Work out the finished part from the listing and answer in its coordinate system (mm). Give positions to 0.01 mm unless a question says otherwise; leave off trailing zeros. Loops run counter-clockwise (first coordinate to the right, second up) from the corner with the lowest first, then second, coordinate; pieces in that order, holes last. Notation, with made-up numbers: (-25.75, -33.75) - (23.25, -33.75) arc R28 ccw to (23.25, 0.25) - close; hole circle Ø11 at (85.25, 5.5). An arc over 180 degrees is marked (long way). Use CSV: the item, a comma, the result in double quotes.
Autodesk Inventor part; units mm, degrees
ref_plane "YZ Plane" through (0, 0, 0) normal (1, 0, 0) x (0, 1, 0)
ref_plane "XZ Plane" through (0, 0, 0) normal (0, 1, 0) x (-1, 0, 0)
ref_plane "XY Plane" through (0, 0, 0) normal (0, 0, 1) x (1, 0, 0)
sketch "Sketch1" plane through (0, 0, 0) normal (0, 0, 1) x (1, 0, 0)
  line L0 (-25, 0) -> (25, 0)
  line L1 (25, 0) -> (25, -1190)
  line L2 (25, -1190) -> (-25, -1190)
  line L3 (-25, -1190) -> (-25, 0)
  line L4 (25, -1190) -> (-25, -1153.2713)
  line L5 (25, 0) -> (-25, -68.0668)
  point P0 (0, 0)
  point P1 (0, 0)
  point P2 (25, -1153.2713)
  dimension "d0" = 50
  dimension "d1" = 1190
  dimension "d5" = 53.7
  dimension "d6" = 53.7
extrude "Plate1" add sketch "Sketch1" along normal mid plane 3 contours L1 L4 L3 L5
chamfer "Corner Chamfer1" distance 3 angle 45 1 edges at (25, -1190, 0)
fillet "Corner Round1" radius 6 1 edges at (-25, -1153.2713, 0)
fillet "Corner Round2" radius 6 1 edges at (-25, -68.0668, 0)
chamfer "Corner Chamfer3" distance 3 angle 45 1 edges at (25, 0, 0)
sketch "Sketch3" plane through (0, 0, 1.5) normal (0, 0, 1) x (1, 0, 0)
  line L0 (-1, -188.5) -> (25, -188.5)
  line L1 (25, -188.5) -> (25, -185.5)
  line L2 (25, -185.5) -> (-1, -185.5)
  line L3 (-1, -185.5) -> (-1, -188.5)
  line L4 (25, -3) -> (25, -1187)
  point P0 (0, 0)
  point P1 (25, -187)
  dimension "d18" = 187
  dimension "d19" = 26
  dimension "d20" = 3
extrude "Extrusion1" cut sketch "Sketch3" against normal through all
pattern_linear "Rectangular Pattern1" count 3 spacing 323 along (0, -1, 0) of "Extrusion1"
sketch "Sketch4" plane through (0, 0, -1.5) normal (0, 0, -1) x (-1, 0, 0)
  line L0 (-5.565, -286.9038) -> (3.4627, -286.9038) construction
  line L1 (3.4627, -286.9038) -> (3.4627, -416.417) construction
  line L2 (3.4627, -416.417) -> (-5.565, -416.417) construction
  line L3 (-5.565, -416.417) -> (-5.565, -286.9038) construction
  point P0 (0, 0)
mark "Mark1"
equation "\"d6\" = d5"
equation "\"d2\" = Thickness"
equation "\"BendReliefWidth\" = Thickness"
equation "\"BendReliefDepth\" = 0.5 * Thickness"
equation "\"CornerReliefSize\" = 4 * Thickness"
equation "\"MinimumRemnant\" = 2 * Thickness"
equation "\"TransitionRadius\" = BendRadius"
equation "\"JacobiRadiusSize\" = BendRadius"
equation "\"GapSize\" = Thickness"
properties part number "MSC 602 STRINGER CONE EXIT BACK" material "Stainless Steel"
Item 1: Find the intervals of material crossed by line 1 (Y direction, x = 19, z = 1.1); line 2 (Y direction, x = 16, z = 0.5); line 3 (Y direction, x = -15, z = 0.3), in increasing order.
Determined:
line 1,"y = -1185.59 to -834.5, -831.5 to -511.5, -508.5 to -188.5, -185.5 to -8.17"
line 2,"y = -1183.39 to -834.5, -831.5 to -511.5, -508.5 to -188.5, -185.5 to -12.25"
line 3,"y = -1160.62 to -54.45"
Item 2: A cutting plane is placed at B-B on z = -0.6. Determine the outline of the cut face in (x, y), and give its area (3 significant figures).
Determined:
outline,"(-25, -1150.23) arc R6 ccw to (-22.55, -1155.07) - (22.58, -1188.22) - (25, -1187) - (25, -834.5) - (-1, -834.5) - (-1, -831.5) - (25, -831.5) - (25, -511.5) - (-1, -511.5) - (-1, -508.5) - (25, -508.5) - (25, -188.5) - (-1, -188.5) - (-1, -185.5) - (25, -185.5) - (25, -3) - (23.22, -2.42) - (-23.84, -66.48) arc R6 ccw to (-25, -70.03) - close"
area,"56,600 mm²"
Item 3: A cutting plane is placed at A-A on x = 11. Determine the outline of the cut face in (y, z), and give its area (3 significant figures).
Determined:
outline,"(-1179.72, -1.5) - (-834.5, -1.5) - (-834.5, 1.5) - (-1179.72, 1.5) - close; (-831.5, -1.5) - (-511.5, -1.5) - (-511.5, 1.5) - (-831.5, 1.5) - close; (-508.5, -1.5) - (-188.5, -1.5) - (-188.5, 1.5) - (-508.5, 1.5) - close; (-185.5, -1.5) - (-19.06, -1.5) - (-19.06, 1.5) - (-185.5, 1.5) - close"
area,"3,450 mm²"
Item 4: Given P1, Ø0.9, axis at x = 17.5, z = 0.5, coming from the -Y side; P2, Ø0.9, axis at x = 16.5, z = 0.5, coming from the -Y side; P3, Ø1.5, axis at x = 17.5, z = 0.5, coming from the +Y side, each flat-ended and moving along its own axis, determine where each tip first touches the part or whether it passes through.
Determined:
P1,"stops at y = -1184.82"
P2,"stops at y = -1184.09"
P3,"stops at y = -9.19"
